```python
from build123d import *

# Parameters (mm, degrees)
BOSS_EXTRUDE1_DEPTH          = 16
CHAMFER2_SIZE                = 2
ENL_V_MAT_EXTRU_1_REACH      = 39.537
ENL_V_MAT_EXTRU_1_END_RADIUS = 3
ESQUISSE1_R                  = 3
ESQUISSE2_W                  = 9.751627811
ESQUISSE2_H                  = 34.282380126
ENL_V_MAT_EXTRU_2_DEPTH      = 56
ENL_V_MAT_EXTRU_3_DEPTH      = 3.3
ENL_V_MAT_EXTRU_3_DEPTH_BACK = 3.3
ESQUISSE8_R                  = 1.5
ENL_V_MAT_EXTRU_4_DEPTH      = 10.3
ESQUISSE9_R                  = 2
ENL_V_MAT_EXTRU_5_DEPTH      = 2
ENL_V_MAT_EXTRU_6_DEPTH      = 7
CONG_1_R                     = 3


with BuildPart() as part:
    # Sketch1 → Boss-Extrude1 (new body)
    with BuildSketch(Plane(origin=(0, 0, 0), x_dir=(0, -1, 0), z_dir=(1, 0, 0))):
        with BuildLine():
            ThreePointArc((-8, 0), (0, 8), (8, 0))
            Line((8, 0), (8, 25))
            Line((8, 25), (-8, 25))
            Line((-8, 25), (-8, 0))
        make_face()
        with BuildLine():
            ThreePointArc((-3, 0), (0, 3), (3, 0))
            Line((3, 0), (8, 0))
            ThreePointArc((8, 0), (0, 8), (-8, 0))
            Line((-8, 0), (-3, 0))
        make_face()
        with BuildLine():
            Line((8, 0), (3, 0))
            ThreePointArc((3, 0), (0, -3), (-3, 0))
            Line((-3, 0), (-8, 0))
            ThreePointArc((-8, 0), (0, -8), (8, 0))
        make_face()
    extrude(amount=BOSS_EXTRUDE1_DEPTH)

    # Chamfer2
    chamfer2_edges = [part.edges().sort_by_distance(p)[0] for p in [
        (16, 8, -12.5),
        (16, 0, 8),
        (0, 8, -12.5),
        (0, -8, -12.5),
        (0, 0, 8),
        (16, -8, -12.5),
    ]]
    chamfer(chamfer2_edges, length=CHAMFER2_SIZE)

    # Enlèv. mat.-Extru.1: up to this cylinder (the profile starts outside it)
    enl_v_mat_extru_1_end = Plane(origin=(8, 0, 0), z_dir=(-1, 0, 0)) * Cylinder(ENL_V_MAT_EXTRU_1_END_RADIUS, 86.074, mode=Mode.PRIVATE)
    # Esquisse1 → Enlèv. mat.-Extru.1 (cut, up to the surface)
    with BuildSketch(Plane(origin=(0, 0, -25), x_dir=(-1, 0, 0), z_dir=(0, 0, -1)), mode=Mode.PRIVATE) as enl_v_mat_extru_1_sk1:
        with Locations((-8, 0)):
            Circle(ESQUISSE1_R)
    enl_v_mat_extru_1_tool1 = extrude(enl_v_mat_extru_1_sk1.sketch, amount=-ENL_V_MAT_EXTRU_1_REACH, mode=Mode.PRIVATE) - enl_v_mat_extru_1_end
    add(enl_v_mat_extru_1_tool1.solids().sort_by_distance((8, 0, -25))[0], mode=Mode.SUBTRACT)

    # Esquisse2 → Enlèv. mat.-Extru.2 (cut)
    with BuildSketch(Plane(origin=(0, 8, 0), x_dir=(1, 0, 0), z_dir=(0, 1, 0))):
        with Locations((12.875813906, 7.858809937)):
            Rectangle(ESQUISSE2_W, ESQUISSE2_H)
    extrude(amount=-ENL_V_MAT_EXTRU_2_DEPTH, mode=Mode.SUBTRACT)

    # Esquisse4 → Enlèv. mat.-Extru.3 (cut, two sides: drawn at the far end of the back side and taken through both)
    with BuildSketch(Plane.XY.offset(-12).offset(-ENL_V_MAT_EXTRU_3_DEPTH_BACK)):
        Polygon((13.196152423, -3), (13.196152423, 3), (8, 6), (2.803847577, 3), (2.803847577, -3), (8, -6), align=None)
    extrude(amount=ENL_V_MAT_EXTRU_3_DEPTH + ENL_V_MAT_EXTRU_3_DEPTH_BACK, mode=Mode.SUBTRACT)

    # Esquisse8 → Enlèv. mat.-Extru.4 (cut)
    with BuildSketch(Plane(origin=(8, 0, 0), x_dir=(0, 0, -1), z_dir=(1, 0, 0))):
        with Locations((6.308944807, 5.5)):
            Circle(ESQUISSE8_R)
        with Locations(Location((6.308944807, -5.5, 0), (0, 0, 340.528779366))):
            Circle(ESQUISSE8_R)
    extrude(amount=-ENL_V_MAT_EXTRU_4_DEPTH, mode=Mode.SUBTRACT)

    # Esquisse9 → Enlèv. mat.-Extru.5 (cut)
    with BuildSketch(Plane.ZY):
        with Locations((-6.308944807, 5.5)):
            Circle(ESQUISSE9_R)
        with Locations(Location((-6.308944807, -5.5, 0), (0, 0, 345.522487814))):
            Circle(ESQUISSE9_R)
    extrude(amount=-ENL_V_MAT_EXTRU_5_DEPTH, mode=Mode.SUBTRACT)

    # Esquisse10 → Enlèv. mat.-Extru.6 (cut)
    with BuildSketch(Plane(origin=(0, 0, -25), x_dir=(-1, 0, 0), z_dir=(0, 0, -1))):
        with BuildLine():
            Line((-8, 8), (-8, 5))
            ThreePointArc((-8, 5), (-3, 0), (-8, -5))
            Line((-8, -5), (-8, -5.041535343))
            Line((-8, -5.041535343), (-8, -8))
            Line((-8, -8), (-2, -8))
            Line((-2, -8), (0, -6))
            Line((0, -6), (0, 6))
            Line((0, 6), (-2, 8))
            Line((-2, 8), (-8, 8))
        make_face()
    extrude(amount=-ENL_V_MAT_EXTRU_6_DEPTH, mode=Mode.SUBTRACT)

    # Congé1
    cong_1_edges = [part.edges().sort_by_distance(p)[0] for p in [
        (5, -8, -18),
        (1, -7, -18),
        (0, 0, -18),
        (1, 7, -18),
        (5, 8, -18),
    ]]
    fillet(cong_1_edges, radius=CONG_1_R - 0.0001)  # a hair under: the kernel refuses the full size


solid = part.part
```
The listing builds one solid part. Answer for the finished solid, in the listing's coordinates (mm). A direction names the side the tool comes from. Give positions to 0.01 mm unless a question says otherwise; leave off trailing zeros. Order: outer loops, then holes, each group sorted by start corner. A loop starts at its lowest first (then second) coordinate and runs counter-clockwise, first axis right, second up.
Item 1: Which of the six approach directions +Z, -Z, +X, -X, +Y, -Y give full straight-line access (tool end or side, diameter ignored) to faces 4 (the face through (5, -8, -7)), 5 (the face through (5, 0, -20)), 6 (the face through (0.986, 3.548, -6.743)), 7 (the face through (0.3, 0.1, 6.3)), 8 (the face through (2.804, 0, -12))?
From the geometry:
face 4: +Z, -Z, +X, -X, -Y
face 5: -Z, +X
face 6: -X
face 7: +Z, -X
face 8: +X
Item 2: The part is cut by section D-D, the plane z = -21. Give the vertices of the cut face in (x, y).
From the geometry:
outline: (8, -5) - (8, -3) arc R3 cw to (8, 3) - (8, 5) arc R5 ccw to start
Item 3: Given pin 1 Ø3 at (x, y) = (2, 5.5) entering from -Z; pin 2 Ø1 at (y, z) = (0, -16.5) entering from +X, each flat-ended and moving along its own axis, determine where each tip first touches the part or whether it passes through.
From the geometry:
pin 1: stops at z = -18
pin 2: stops at x = 5.04
Item 4: The part is cut by section B-B, the plane z = -6.5. Give the vertices of the cut face in (x, y), and give its area (3 significant figures).
From the geometry:
outline: (0, -3.51) - (2, -3.51) - (2, -4.01) - (8, -4.01) - (8, -3) arc R3 cw to (8, 3) - (8, 4.01) - (2, 4.01) - (2, 3.51) - (0, 3.51) - close; (1.49, -7.49) - (2, -8) - (8, -8) - (8, -6.99) - (2, -6.99) - (2, -7.49) - close; (1.49, 7.49) - (2, 7.49) - (2, 6.99) - (8, 6.99) - (8, 8) - (2, 8) - close
area: 60.5 mm2
Item 5: For a pull along Y with two mould halves and no side action, classify faces 1 (the face through (3, 0, -22)), 2 (the face through (8, -3.4, -4.6)), 3 (the face through (5.04, -6.77, -5.51)) as pulls with the +Y half, pulls with the -Y half, needs draft (parallel to the pull), parting line crosses it, or undercut.
From the geometry:
face 1: parting line crosses it
face 2: needs draft
face 3: undercut
Item 6: Find the intervals of material crossed by probe 1 along Z at (x, y) = (4, -2.75); probe 2 along Y at (x, z) = (4.75, -6.5); probe 3 along Y at (x, z) = (2.75, -2), in increasing order.
From the geometry:
probe 1: z = -25 to -15.3, -8.7 to -1.2, 1.2 to 7.51
probe 2: y = -8 to -6.99, -4.01 to 4.01, 6.99 to 8
probe 3: y = -8 to -2.24, 2.24 to 8
Item 7: The part is cut by section C-C, the plane x = 6. Give the vertices of the cut face in (y, z).
From the geometry:
outline: (-8, -15) arc R3 ccw to (-5, -18) - (-4.58, -18) - (-4.58, -25) - (-2.24, -25) - (-2.24, -15.3) - (-4.85, -15.3) - (-4.85, -8.7) - (-2.24, -8.7) - (-2.24, -2) arc R3 cw (long way) to (2.24, -2) - (2.24, -8.7) - (4.85, -8.7) - (4.85, -15.3) - (2.24, -15.3) - (2.24, -25) - (4.58, -25) - (4.58, -18) - (5, -18) arc R3 ccw to (8, -15) - (8, 0) arc R8 ccw to (-8, 0) - close; hole circle Ø3 at (-5.5, -6.31); hole circle Ø3 at (5.5, -6.31)
